```python
from build123d import *

# Parameters (mm, degrees)
EXTRUDE_1_DEPTH     = 8
SKETCH_2_R          = 1.05
CUT_EXTRUDE_1_DEPTH = 10.283823749
CHAMFER_1_SIZE      = 0.25


with BuildPart() as part:
    # ｽｹｯﾁ1 → ﾎﾞｽ - 押し出し1 (new body)
    with BuildSketch(Plane.XY):
        Polygon((-3.507584264, 0), (-1.492415736, 0), (-1.007584264, -1.2), (1.007584264, -1.2), (1.492415736, 0), (3.507584264, 0), (3.992415736, -1.2), (3.992415736, -2.5), (-3.992415736, -2.5), (-3.992415736, -1.2), align=None)
    extrude(amount=EXTRUDE_1_DEPTH)

    # ｽｹｯﾁ2 → ｶｯﾄ - 押し出し1 (cut, through all)
    with BuildSketch(Plane.XZ.offset(2.5)):
        with Locations((0, 4)):
            Circle(SKETCH_2_R)
    extrude(amount=-CUT_EXTRUDE_1_DEPTH, mode=Mode.SUBTRACT)

    # ｽｹｯﾁ4 → ｶｯﾄ - 回転1 (revolve, cut)
    with BuildSketch(Plane(origin=(0, 0, 0), x_dir=(0, 0, -1), z_dir=(1, 0, 0))):
        Polygon((-4, -2.5), (-2, -2.5), (-2, -2.3), (-3, -1.3), (-4, -1.3), align=None)
    revolve(axis=Axis((0, -2.5, 4), (0, 1, 0)), mode=Mode.SUBTRACT)

    # 面取り1
    chamfer_1_edges = [part.edges().sort_by_distance(p)[0] for p in [
        (3.992415736, -2.5, 4),
        (-3.992415736, -2.5, 4),
        (0, -2.5, 8),
        (0, -2.5, 0),
    ]]
    chamfer(chamfer_1_edges, length=CHAMFER_1_SIZE)


solid = part.part
```
The listing builds one solid part. Answer for the finished solid, in the listing's coordinates (mm). A direction names the side the tool comes from. Give positions to 0.01 mm unless a question says otherwise; leave off trailing zeros. Order: outer loops, then holes, each group sorted by start corner. A loop starts at its lowest first (then second) coordinate and runs counter-clockwise, first axis right, second up. Notation, with made-up numbers: M 79,20.5 L 96,20.5 A16 cw 96,35.5 Z; hole C 20.5,-28.75 d3. An arc over 180 degrees is marked long. Put each result on its own line as item: value. Start each with the question number.
Item 1: Find the intervals of material crossed by line 1 along X through (y, z) = (-1.25, 4); line 2 along Z through (x, y) = (0, -1.3); line 3 along X through (y, z) = (-2.05, 5.5), in increasing order.
Item 2: The part is cut by section C-C, the plane y = -0.55. Determine the outline of the cut face in (x, z), and give its area (3 significant figures).
Item 3: The part is cut by section A-A, the plane x = 0. Determine the outline of the cut face in (y, z), and give its area (4 significant figures).
Item 4: Which of the six approach directions +Z, -Z, +X, -X, +Y, -Y give full straight-line access (tool end or side, diameter ignored) to faces 1 (the face through (0, -1.2, 1)), 2 (the face through (-3, 0, 4))?
Item 5: For a pull along X with two mould halves and no side action, classify faces 3 (the face through (0.1, -1.4, 8)), 4 (the face through (3.747, -0.592, 3.944)), 5 (the face through (-1.253, -0.592, 3.944)), 6 (the face through (0, -1.2, 7)) as +X half, -X half, draft (parallel to the pull), parting line (faces both ways), or undercut.
Item 6: A flat-ended cylindrical pin translates along its axis: P1, Ø1.6, axis at x = 0, z = 5.5, coming from the +Y side. Find the tip coordinate at first contact, or state that the pin passes through.
Item 7: The part is cut by section D-D, the plane z = 7. Determine the outline of the cut face in (x, y).
Item 8: The part is cut by section B-B, the plane z = 4. Determine the outline of the cut face in (x, y).
Answer key:
1. line 1: x = -3.99 to -1.05, 1.05 to 3.99
1. line 2: z = 0 to 2.95, 5.05 to 8
1. line 3: x = -3.99 to -0.9, 0.9 to 3.99
2. outline: M -3.73,0 L -1.27,0 L -1.27,8 L -3.73,8 Z; M 1.27,0 L 3.73,0 L 3.73,8 L 1.27,8 Z
2. area: 39.4 mm²
3. outline: M -2.5,0.25 L -2.25,0 L -1.2,0 L -1.2,2.95 L -1.35,2.95 L -2.3,2 L -2.5,2 Z; M -2.5,6 L -2.3,6 L -1.35,5.05 L -1.2,5.05 L -1.2,8 L -2.25,8 L -2.5,7.75 Z
3. area: 6.325 mm²
4. face 1: +Z, -Z, +Y
4. face 2: +Z, -Z, +X, -X, +Y
5. face 3: draft
5. face 4: +X half
5. face 5: undercut
5. face 6: undercut
6. P1: stops at y = -1.2
7. outline: M -3.99,-2.25 L -3.74,-2.5 L 3.74,-2.5 L 3.99,-2.25 L 3.99,-1.2 L 3.51,0 L 1.49,0 L 1.01,-1.2 L -1.01,-1.2 L -1.49,0 L -3.51,0 L -3.99,-1.2 Z
8. outline: M -3.99,-2.25 L -3.74,-2.5 L -2,-2.5 L -2,-2.3 L -1.05,-1.35 L -1.05,-1.1 L -1.49,0 L -3.51,0 L -3.99,-1.2 Z; M 1.05,-1.35 L 2,-2.3 L 2,-2.5 L 3.74,-2.5 L 3.99,-2.25 L 3.99,-1.2 L 3.51,0 L 1.49,0 L 1.05,-1.1 Z
